The model under review builds one solid part; all positions refer to its coordinate system, in mm. Face numbers are marked on the shaded views. Round coordinates to 2 decimals unless told otherwise and drop trailing zeros. Write each loop counter-clockwise with the first axis right and the second up, starting at its lowest first coordinate (ties: lowest second). Pieces come first, ordered by that corner, then holes.
Item 1: Add section A-A (y = 57). Give the boundary of the cut face in (x, z).
Item 2: Add section C-C (z = 5.5). Give the boundary of the cut face in (x, y).
Item 3: To check wall thickness, follow L1, parallel to Y at x = 36, z = 7.5; L2, parallel to X at y = 32, z = 6.25; L3, parallel to X at y = 66, z = 3.75. State the ranges of each line that lie inside material, in increasing order.
Item 4: Draft analysis for pull direction X (two halves, no side actions). For the marked faces 1, 2, 3 and 4, state which applies: +X half, -X half, draft (parallel to the pull), parting line (faces both ways), or undercut.
Item 5: Add section B-B (x = 20). Give the boundary of the cut face in (y, z), plus the area to 4 significant figures.
Item 6: Clearance check with flat-ended pins moving along their axes: pin 1 Ø1.6 at (x, z) = (-12.5, 6) entering from +Y; pin 2 Ø5 at (x, y) = (-7.76, 33.41) entering from +Z; pin 3 Ø0.6 at (x, z) = (-12.5, 6) entering from -Y; pin 4 Ø2.5 at (x, y) = (-7.76, 64.41) entering from -Z. State where each tip first meets the part, or that it passes through.
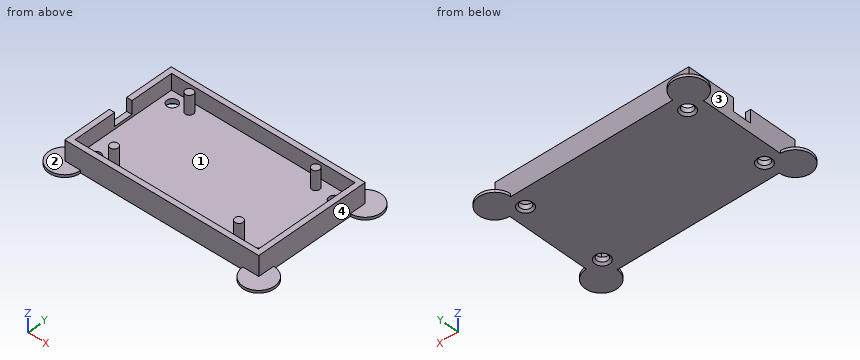
```python
from build123d import *

# Parameters (mm, degrees)
F0_R           = 2
F0_R_2         = 1.5
F0_W           = 2
F0_H           = 7
F1_DEPTH       = 2.5
F2_DEPTH       = 8.5
F3_DEPTH       = 9.6
F4_DEPTH       = 3.5
F5_D           = 3
F5_CSINK_D     = 5.5
F5_CSINK_ANGLE = 90
F6_DEPTH       = 1


with BuildPart() as f1:
    # F0 (on Top) → F1 (new body)
    with BuildSketch(Plane.XY):
        Polygon((57.2425711751, 68.4110085815), (-11.7574288249, 68.4110085815), (-11.7574288249, 52.4110085815), (-11.7574288249, 45.4110085815), (-11.7574288249, 29.4110085815), (57.2425711751, 29.4110085815), align=None)
        with Locations((-7.7574288249, 33.4110085815)):
            Circle(F0_R, mode=Mode.SUBTRACT)
        with Locations((-1.2574288249, 33.9110085815)):
            Circle(F0_R_2, mode=Mode.SUBTRACT)
        with Locations((45.7425711751, 33.9110085815)):
            Circle(F0_R_2, mode=Mode.SUBTRACT)
        with Locations((53.2425711751, 33.4110085815)):
            Circle(F0_R, mode=Mode.SUBTRACT)
        with Locations((-7.7574288249, 64.4110085815)):
            Circle(F0_R, mode=Mode.SUBTRACT)
        with Locations((-1.8220887287, 64.9110085815)):
            Circle(F0_R_2, mode=Mode.SUBTRACT)
        with Locations((45.7425711751, 64.9110085815)):
            Circle(F0_R_2, mode=Mode.SUBTRACT)
        with Locations((53.2425711751, 64.4110085815)):
            Circle(F0_R, mode=Mode.SUBTRACT)
        Polygon((-11.7574288249, 52.4110085815), (-11.7574288249, 68.4110085815), (57.2425711751, 68.4110085815), (57.2425711751, 29.4110085815), (-11.7574288249, 29.4110085815), (-11.7574288249, 45.4110085815), (-13.7574288249, 45.4110085815), (-13.7574288249, 33.4110085815), (-13.7574288249, 27.4110085815), (-7.7574288249, 27.4110085815), (53.2425711751, 27.4110085815), (59.2425711751, 27.4110085815), (59.2425711751, 33.4110085815), (59.2425711751, 64.4110085815), (59.2425711751, 70.4110085815), (53.2425711751, 70.4110085815), (-7.7574288249, 70.4110085815), (-13.7574288249, 70.4110085815), (-13.7574288249, 64.4110085815), (-13.7574288249, 52.4110085815), align=None)
        with Locations((-1.2574288249, 33.9110085815)):
            Circle(F0_R_2)
        with Locations((45.7425711751, 33.9110085815)):
            Circle(F0_R_2)
        with Locations((45.7425711751, 64.9110085815)):
            Circle(F0_R_2)
        with Locations((-1.8220887287, 64.9110085815)):
            Circle(F0_R_2)
        with Locations((-12.7574288249, 48.9110085815)):
            Rectangle(F0_W, F0_H)
    extrude(amount=F1_DEPTH)

    # F0 (on Top) → F2 (join)
    with BuildSketch(Plane.XY):
        Polygon((-11.7574288249, 52.4110085815), (-11.7574288249, 68.4110085815), (57.2425711751, 68.4110085815), (57.2425711751, 29.4110085815), (-11.7574288249, 29.4110085815), (-11.7574288249, 45.4110085815), (-13.7574288249, 45.4110085815), (-13.7574288249, 33.4110085815), (-13.7574288249, 27.4110085815), (-7.7574288249, 27.4110085815), (53.2425711751, 27.4110085815), (59.2425711751, 27.4110085815), (59.2425711751, 33.4110085815), (59.2425711751, 64.4110085815), (59.2425711751, 70.4110085815), (53.2425711751, 70.4110085815), (-7.7574288249, 70.4110085815), (-13.7574288249, 70.4110085815), (-13.7574288249, 64.4110085815), (-13.7574288249, 52.4110085815), align=None)
    extrude(amount=F2_DEPTH)

    # F0 (on Top) → F3 (join)
    with BuildSketch(Plane.XY):
        with Locations((-1.8220887287, 64.9110085815)):
            Circle(F0_R_2)
        with Locations((-1.2574288249, 33.9110085815)):
            Circle(F0_R_2)
        with Locations((45.7425711751, 33.9110085815)):
            Circle(F0_R_2)
        with Locations((45.7425711751, 64.9110085815)):
            Circle(F0_R_2)
    extrude(amount=F3_DEPTH)

    # F0 (on Top) → F4 (join)
    with BuildSketch(Plane.XY):
        with Locations((-12.7574288249, 48.9110085815)):
            Rectangle(F0_W, F0_H)
    extrude(amount=F4_DEPTH)

    # F5 (through all)
    with Locations(Plane(origin=(0, 0, 0), x_dir=(1, 0, 0), z_dir=(0, 0, -1))):
        with Locations((53.2425711751, -64.4110085815), (53.2425711751, -33.4110085815), (-7.7574288249, -33.4110085815), (-7.7574288249, -64.4110085815)):
            CounterSinkHole(F5_D / 2, F5_CSINK_D / 2, counter_sink_angle=F5_CSINK_ANGLE)

    # F0 (on Top) → F6 (join)
    with BuildSketch(Plane.XY):
        with BuildLine():
            ThreePointArc((-7.7574288249, 70.4110085815), (-18.000069512, 74.6536492686), (-13.7574288249, 64.4110085815))
            Line((-13.7574288249, 64.4110085815), (-13.7574288249, 70.4110085815))
            Line((-13.7574288249, 70.4110085815), (-7.7574288249, 70.4110085815))
        make_face()
        with BuildLine():
            ThreePointArc((59.2425711751, 64.4110085815), (63.4852118622, 74.6536492686), (53.2425711751, 70.4110085815))
            Line((53.2425711751, 70.4110085815), (59.2425711751, 70.4110085815))
            Line((59.2425711751, 70.4110085815), (59.2425711751, 64.4110085815))
        make_face()
        with BuildLine():
            Line((59.2425711751, 27.4110085815), (53.2425711751, 27.4110085815))
            ThreePointArc((53.2425711751, 27.4110085815), (63.4852118622, 23.1683678944), (59.2425711751, 33.4110085815))
            Line((59.2425711751, 33.4110085815), (59.2425711751, 27.4110085815))
        make_face()
        with BuildLine():
            Line((-13.7574288249, 27.4110085815), (-13.7574288249, 33.4110085815))
            ThreePointArc((-13.7574288249, 33.4110085815), (-18.000069512, 23.1683678944), (-7.7574288249, 27.4110085815))
            Line((-7.7574288249, 27.4110085815), (-13.7574288249, 27.4110085815))
        make_face()
    extrude(amount=F6_DEPTH)


solid = f1.part
```
Numbers:
1. outline: (-13.76, 0) - (59.24, 0) - (59.24, 8.5) - (57.24, 8.5) - (57.24, 2.5) - (-11.76, 2.5) - (-11.76, 8.5) - (-13.76, 8.5) - close
2. outline: (-13.76, 27.41) - (59.24, 27.41) - (59.24, 70.41) - (-13.76, 70.41) - (-13.76, 52.41) - (-11.76, 52.41) - (-11.76, 68.41) - (57.24, 68.41) - (57.24, 29.41) - (-11.76, 29.41) - (-11.76, 45.41) - (-13.76, 45.41) - close; circle Ø3 at (-1.82, 64.91); circle Ø3 at (-1.26, 33.91); circle Ø3 at (45.74, 33.91); circle Ø3 at (45.74, 64.91)
3. L1: y = 27.41 to 29.41, 68.41 to 70.41
3. L2: x = -13.76 to -11.76, 57.24 to 59.24
3. L3: x = -13.76 to -11.76, -2.85 to -0.79, 44.71 to 46.77, 57.24 to 59.24
4. face 1: undercut
4. face 2: draft
4. face 3: -X half
4. face 4: +X half
5. outline: (27.41, 0) - (70.41, 0) - (70.41, 8.5) - (68.41, 8.5) - (68.41, 2.5) - (29.41, 2.5) - (29.41, 8.5) - (27.41, 8.5) - close
5. area: 131.5 mm2
6. pin 1: stops at y = 70.41
6. pin 2: stops at z = 2.5
6. pin 3: stops at y = 27.41
6. pin 4: passes through
